Read the model definition and answer for the solid it produces. Units are mm, in the model's axes. Face numbers are marked on the shaded views. A direction names the side the tool comes from. Give positions to 0.01 mm unless a question says otherwise; leave off trailing zeros. Order: outer loops, then holes, each group sorted by start corner. A loop starts at its lowest first (then second) coordinate and runs counter-clockwise, first axis right, second up. Notation, with made-up numbers: (-19, 44) - (30, 44) arc R17 cw to (30, 66) - close; hole circle Ø9 at (-27.5, -23.5). An arc over 180 degrees is marked (long way). Return JSON: item names as keys, results as strings.
```python
from build123d import *

# Parameters (mm, degrees)
F1_DEPTH      = 12.5
F1_DEPTH_BACK = 12.5
F4_DEPTH      = 4.5
F5_R          = 10
F6_R          = 4
F7_R          = 3
F8_R          = 1


# Not quite as in the source:
# - a pattern or mirror of a feature is missing from the dataset's text; its kind, count and spacing are read off the source's solid


with BuildPart() as f1:
    # F0 (on Front) → F1 (new body, two sides)
    with BuildSketch(Plane.XZ) as f1_sk:
        Polygon((0, 5), (0, 0), (70, 0), (70, 5), (38.7070253131, 15), (55.1869723842, 43.5441056332), (41.7811946296, 54.7928888027), align=None)
    extrude(amount=F1_DEPTH)
    extrude(f1_sk.sketch, amount=-F1_DEPTH_BACK)

    # F3 (on offset) → F4 (cut)
    with BuildSketch(Plane.XZ.offset(3)):
        with BuildLine():
            Line((52.8888390549, 45.4724684623), (44.079327959, 52.8645259737))
            Line((44.079327959, 52.8645259737), (8.0516093002, 9.9283628291))
            ThreePointArc((8.0516093002, 9.9283628291), (7.6308192684, 6.7321452148), (10.3497426295, 5))
            Line((10.3497426295, 5), (11.933790823, 5))
            ThreePointArc((11.933790823, 5), (18.2730647491, 6.4053831945), (23.4244574698, 10.3581858547))
            Line((23.4244574698, 10.3581858547), (52.8888390549, 45.4724684623))
        make_face()
    f4 = extrude(amount=F4_DEPTH, mode=Mode.SUBTRACT)

    # F4_copies: F4 across plane
    add(f4.mirror(Plane.ZX), mode=Mode.SUBTRACT)

    # F5
    f5_edges = [f1.edges().sort_by_distance(p)[0] for p in [
        (38.707025, 0, 15),
        (0, 0, 5),
    ]]
    fillet(f5_edges, radius=F5_R)

    # F6
    f6_edges = [f1.edges().sort_by_distance(p)[0] for p in [
        (70, 0, 5),
    ]]
    fillet(f6_edges, radius=F6_R)

    # F7
    f7_edges = [f1.edges().sort_by_distance(p)[0] for p in [
        (22.060375, -12.5, 31.290531),
        (50.049611, -12.5, 34.645935),
        (50.049611, 12.5, 34.645935),
        (22.060375, 12.5, 31.290531),
        (70, -12.5, 1.039484),
        (69.230351, -12.5, 4.437958),
        (58.873064, -12.5, 8.55573),
        (0, -12.5, 0.680149),
        (44.245427, -12.5, 17.141433),
        (0.603074, -12.5, 4.780499),
        (70, 12.5, 1.039484),
        (69.230351, 12.5, 4.437958),
        (58.873064, 12.5, 8.55573),
        (0, 12.5, 0.680149),
        (44.245427, 12.5, 17.141433),
        (0.603074, 12.5, 4.780499),
    ]]
    fillet(f7_edges, radius=F7_R)

    # F8
    f8_edges = [f1.edges().sort_by_distance(p)[0] for p in [
        (55.186972, 0, 43.544106),
        (54.497154, -11.629423, 44.122932),
        (54.497154, 11.629423, 44.122932),
        (48.466357, -12.5, 49.183371),
        (48.466357, 12.5, 49.183371),
        (42.454302, -11.62132, 54.228084),
        (42.454302, 11.62132, 54.228084),
        (41.781195, 0, 54.792889),
        (52.888839, -5.25, 45.472468),
        (48.484084, -3, 49.168497),
        (48.484084, -7.5, 49.168497),
        (44.079328, -5.25, 52.864526),
        (48.484084, 3, 49.168497),
        (44.079328, 5.25, 52.864526),
        (48.484084, 7.5, 49.168497),
        (52.888839, 5.25, 45.472468),
    ]]
    fillet(f8_edges, radius=F8_R)


solid = f1.part
```
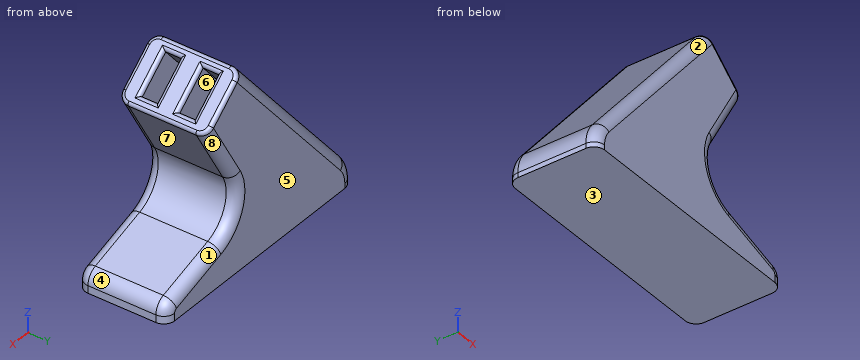
Q1. Given pin 1 (8 mm diameter, centred on x = 10.5, y = -2, fed in from +Z); pin 2 (5 mm diameter, centred on y = 4, z = 10, fed in from -X); pin 3 (2 mm diameter, centred on x = 50.5, y = -6, fed in from +Z); pin 4 (13.5 mm diameter, centred on x = 21, z = 27.5, fed in from -Y), each flat-ended and moving along its own axis, determine where each tip first touches the part or whether it passes through.
Values:
{"pin 1": "stops at z = 22.28", "pin 2": "stops at x = 2.11", "pin 3": "stops at z = 43.82", "pin 4": "stops at y = -12.5"}
Q2. A cutting plane is placed at B-B (x = 26). Give the number of separate pieces and of enclosed holes in the cut face, and give its area (3 significant figures).
Values:
{"separate pieces": "1", "enclosed holes": "2", "area": "733 mm²"}
Q3. A cutting plane is placed at A-A (y = 0). Write down the section's boundary in (x, z).
Values:
{"outline": "(0, 0) - (70, 0) - (70, 2.08) arc R4 ccw to (67.22, 5.89) - (50.53, 11.22) arc R10 cw to (44.91, 25.75) - (54.77, 42.82) arc R1 ccw to (54.54, 44.08) - (42.55, 54.15) arc R1 ccw to (41.14, 54.03) - (2.34, 7.79) arc R10 ccw to (0, 1.36) - close"}
Q4. Determine the mould class of the marked faces 1, 2 and 3 for opening direction Z: released by +Z, released by -Z, zero draft, split by the parting line, or undercut.
Values:
{"face 1": "undercut", "face 2": "released by +Z", "face 3": "released by -Z"}
Q5. Consider L1, parallel to X at y = -7, z = 16.5; L2, parallel to Z at x = 39.5, y = -7; L3, parallel to X at y = 6.5, z = 34. Determine where each line is inside the solid, lowest interval first.
Values:
{"L1": "x = 9.65 to 13.57, 28.58 to 44.52", "L2": "z = 0 to 29.52, 47.41 to 52.07", "L3": "x = 24.33 to 28.25, 43.26 to 49.68"}
Q6. For the marked faces 4, 5, 6, 7 and 8, determine the directions among +Z, -Z, +X, -X, +Y, -Y from which every point of the face is accessible in a straight line to the end or side of a thin tool.
Values:
{"face 4": "+Z, +X, +Y, -Y", "face 5": "+Z, -Z, +X, -X, +Y", "face 6": "none", "face 7": "+X, +Y, -Y", "face 8": "+X, +Y"}
